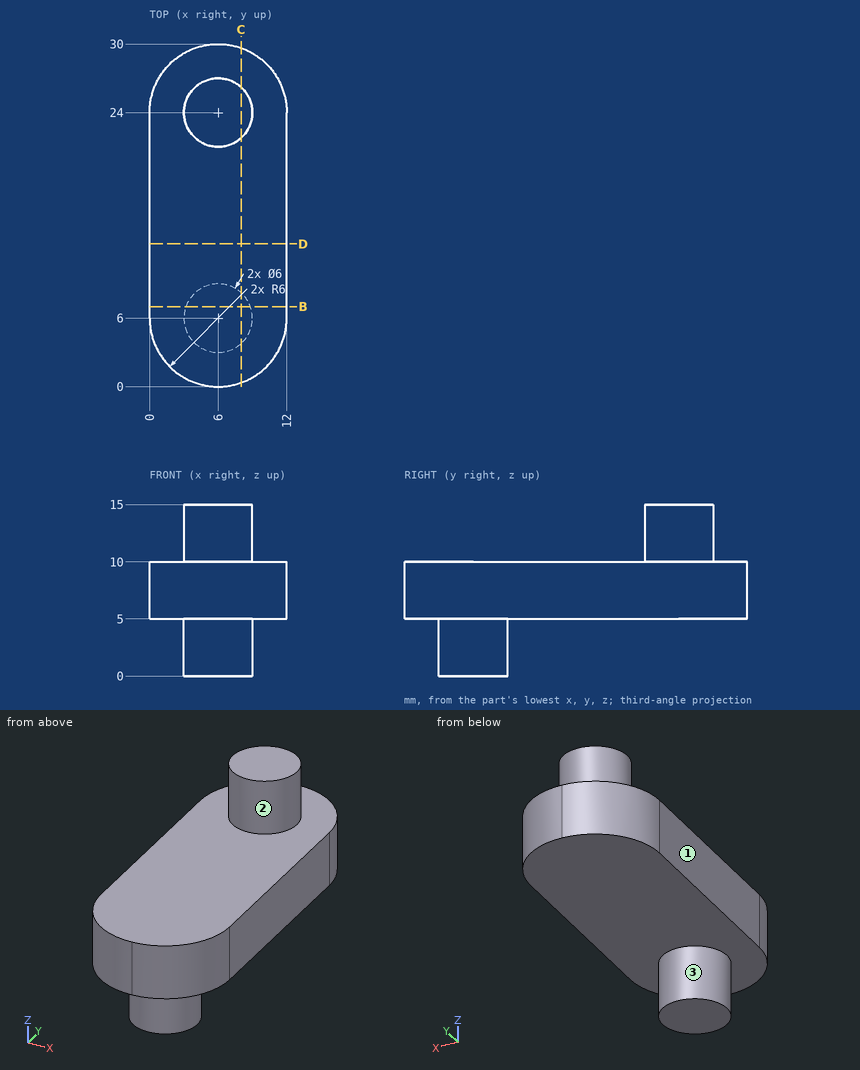
Job drawing, mm, ordinate dimensions from the low corner. One solid piece. A direction names the side the tool comes from. Give positions to 0.01 mm unless a question says otherwise; leave off trailing zeros. Loops run counter-clockwise (first coordinate to the right, second up) from the corner with the lowest first, then second, coordinate; pieces in that order, holes last. Notation, with made-up numbers: (82, 80.25) -> (138, 80.25) arc R24 cw to (138, 112.25) -> close; hole circle Ø8 at (34.25, -4). An arc over 180 degrees is marked (long way). Write each question's results on one line, items separated by ' | '.
(1) Tool access for the marked faces 1, 2 and 3: list every direction of +Z, -Z, +X, -X, +Y, -Y with a clear straight run to the whole face (end or side of a thin tool).
Geometry results:
face 1: +Z, -Z, -X, +Y, -Y | face 2: +Z | face 3: -Z
(2) Cut at C-C on x = 8. List the corners of the cut face in (y, z).
Geometry results:
outline: (0.34, 5) -> (3.76, 5) -> (3.76, 0) -> (8.24, 0) -> (8.24, 5) -> (29.66, 5) -> (29.66, 10) -> (26.24, 10) -> (26.24, 15) -> (21.76, 15) -> (21.76, 10) -> (0.34, 10) -> close
(3) Flat gauge pins, fed straight in: pin 1 Ø3.5 at (x, y) = (4, 11.5) entering from -Z; pin 2 Ø6 at (x, z) = (1.5, 6.5) entering from +Y; pin 3 Ø1.5 at (x, z) = (7, 6.5) entering from -Y. Where does each tip first touch, or does it go through?
Geometry results:
pin 1: stops at z = 5 | pin 2: stops at y = 29.81 | pin 3: stops at y = 0.01
(4) Cut at D-D on y = 12.5. List the corners of the cut face in (x, z).
Geometry results:
outline: (0, 5) -> (12, 5) -> (12, 10) -> (0, 10) -> close
(5) Probe line 1 along Z through (x, y) = (11, 23); line 2 along Z through (x, y) = (7, 5.5); line 3 along Y through (x, z) = (4, 6.75). List the from-to ranges inside material, lowest first.
Geometry results:
line 1: z = 5 to 10 | line 2: z = 0 to 10 | line 3: y = 0.34 to 29.66
(6) Cut at B-B on y = 7. List the corners of the cut face in (x, z), and give its area (3 significant figures).
Geometry results:
outline: (0, 5) -> (3.17, 5) -> (3.17, 0) -> (8.83, 0) -> (8.83, 5) -> (12, 5) -> (12, 10) -> (0, 10) -> close | area: 88.3 mm²
